```python
from build123d import *

# Parameters (mm, degrees)
ZKOSEN_1_SIZE       = 0.5
SKETCH_1_R          = 8.79999935
CUT_EXTRUDE_1_DEPTH = 21


with BuildPart() as part:
    # Skica1 → Rotovat1 (revolve)
    with BuildSketch(Plane.XY, mode=Mode.PRIVATE) as rotovat1_sk:
        Polygon((0, 4.3), (0, 4.175), (45, 4.175), (45, 4.3), (44.3, 4.3), (44.3, 6.3), (45, 6.3), (45, 7.5), (40, 7.5), (40, 7.18), (39, 7.18), (39, 7.5), (6, 7.5), (6, 7.18), (5, 7.18), (5, 7.5), (0, 7.5), (0, 6.3), (0.7, 6.3), (0.7, 4.3), align=None)
    revolve(rotovat1_sk.sketch.rotate(Axis((0, 0, 0), (1, 0, 0)), 90), axis=Axis((0, 0, 0), (1, 0, 0)))

    # Zkosení1
    zkosen_1_edges = [part.edges().sort_by_distance(p)[0] for p in [
        (0, 0, -7.5),
        (45, 0, -7.5),
    ]]
    chamfer(zkosen_1_edges, length=ZKOSEN_1_SIZE)

    # 草图1 → 切除-拉伸1 (cut)
    with BuildSketch(Plane.ZY):
        Circle(SKETCH_1_R)
    extrude(amount=-CUT_EXTRUDE_1_DEPTH, mode=Mode.SUBTRACT)


solid = part.part
```
Here's how the part is built. I have some questions about the finished solid (model axes, mm). A direction names the side the tool comes from. Give positions to 0.01 mm unless a question says otherwise; leave off trailing zeros. Loops run counter-clockwise (first coordinate to the right, second up) from the corner with the lowest first, then second, coordinate; pieces in that order, holes last. Notation, with made-up numbers: M -20.75,31 L 8.25,31 A20 cw 8.25,51 Z; hole C 14.5,44 d2. An arc over 180 degrees is marked long. Put each result on its own line as item: value. Start each with the question number.
(1) For faces 4 (the flat face through (44.3, 4, -3)), 5 (the flat face through (45, -3, 6)), which set-ups out of +Z, -Z, +X, -X, +Y, -Y let a thin tool reach every point of the face, with its end or its side?
(2) Will these pins go through, and if not, where does the flat tip stop? pin 1 Ø6.5 at (y, z) = (-3, 0) entering from +X; pin 2 Ø4 at (x, y) = (31, 3) entering from -Z; pin 3 Ø1.5 at (x, y) = (35.5, -5.5) entering from -Z; pin 4 Ø4 at (x, z) = (26, -4) entering from -Y.
(3) I need wall thicknesses on line 1 along X through (y, z) = (-0.5, 6); line 2 along Z through (x, y) = (42.75, 2); line 3 along Y through (x, z) = (23.5, 3.5). Which ranges of each line are inside material? Lowest first, please. Write a range as [from, to].
(4) I want a section at C-C on x = 35.5. Please give me the cut outline in (y, z) (3 decimals).
(5) I want a section at A-A on z = 0. Please give me the cut outline in (x, y) (3 decimals).
(6) If we mould it in two halves opening along Y, with no side actions, what happens to faces 1 (the flat face through (21, -3.2, 3.2)), 2 (the cylindrical face through (39.49, 6.37, 3.31)), 3 (the cylindrical face through (44.65, 3.83, -5))? For each: +Y half, -Y half, draft (parallel to the pull), parting line (faces both ways), or undercut.
Answer block:
1. face 4: +X
1. face 5: +Z, -Z, +X, +Y, -Y
2. pin 1: x = 45
2. pin 2: z = -7.43
2. pin 3: z = -5.8
2. pin 4: y = -7.23
3. line 1: [21, 44.3]
3. line 2: [-7.23, -3.66], [3.66, 7.23]
3. line 3: [-6.63, -2.28], [2.28, 6.63]
4. outline: C 0,0 d15; hole C 0,0 d8.35
5. outline: M 21,-7.5 L 39,-7.5 L 39,-7.18 L 40,-7.18 L 40,-7.5 L 44.5,-7.5 L 45,-7 L 45,-6.3 L 44.3,-6.3 L 44.3,-4.3 L 45,-4.3 L 45,-4.175 L 21,-4.175 Z; M 21,4.175 L 45,4.175 L 45,4.3 L 44.3,4.3 L 44.3,6.3 L 45,6.3 L 45,7 L 44.5,7.5 L 40,7.5 L 40,7.18 L 39,7.18 L 39,7.5 L 21,7.5 Z
6. face 1: draft
6. face 2: parting line
6. face 3: undercut
